from build123d import *

# Parameters (mm, degrees)
EXTRUDE006_DEPTH                          = 7.5
SKETCH004_R                               = 3.5
EXTRUDE005_DEPTH                          = 10
SKETCH003_AS_DRAWN_R                      = 2.05
EXTRUDE004_DEPTH                          = 4
EXTRUDE004_ONTO_SKETCH003_PLACEMENT_ANGLE = 25.679232
SKETCH002_AS_DRAWN_R                      = 2.05
EXTRUDE003_DEPTH                          = 4
EXTRUDE003_ONTO_SKETCH002_PLACEMENT_ANGLE = 25.679232
EXTRUDE002_DEPTH                          = 3
EXTRUDE001_DEPTH                          = 3
EXTRUDE_DEPTH                             = 100


with BuildPart() as extrude006:
    # Sketch005 (on Face9 of Cut002) → Extrude006 (new body, symmetric)
    with BuildSketch(Plane.XY.offset(-2.969462)):
        Polygon((9.788822, -17.287546), (13.381697, -21.769908), (23.066011, -14.007366), (19.473136, -9.525003), align=None)
        Polygon((74.935691, -52.555563), (78.706554, -57.139857), (89.207015, -48.502584), (85.436152, -43.91829), align=None)
        Polygon((9.274179, -44.439739), (14.585862, -39.004322), (26.329694, -50.48081), (21.018012, -55.916228), align=None)
        Polygon((69.684992, -9.981081), (73.170384, -6.034964), (84.857305, -16.35739), (81.371913, -20.303507), align=None)
    extrude(amount=EXTRUDE006_DEPTH, both=True)


with BuildPart() as extrude005:
    # Sketch004 (on Face13 of Cut001) → Extrude005 (new body, symmetric)
    with BuildSketch(Plane(origin=(0, 2.547184, 0), x_dir=(-1, 0, 0), z_dir=(0, 1, 0))):
        with Locations((-25.011261, 6.853597)):
            Circle(SKETCH004_R)
    extrude(amount=EXTRUDE005_DEPTH, both=True)


with BuildPart() as extrude004:
    # Sketch003 as drawn → Extrude004 (new)
    with BuildSketch(Plane.XY):
        with Locations((6.469403, -53.574993)):
            Circle(SKETCH003_AS_DRAWN_R)
        with Locations((93.253448, -53.665895)):
            Circle(SKETCH003_AS_DRAWN_R)
    extrude(amount=-EXTRUDE004_DEPTH)


with BuildPart() as extrude004_1:
    # Extrude004 onto Sketch003 placement: moved
    add(extrude004.part.moved(Location((0, -14.53972, 30.239351))).rotate(Axis((0, -14.53972, 30.239351), (1, 0, 0)), EXTRUDE004_ONTO_SKETCH003_PLACEMENT_ANGLE))


with BuildPart() as extrude003:
    # Sketch002 as drawn → Extrude003 (new)
    with BuildSketch(Plane.XY):
        with Locations((7.867664, 15.865227)):
            Circle(SKETCH002_AS_DRAWN_R)
        with Locations((92.333176, 15.993219)):
            Circle(SKETCH002_AS_DRAWN_R)
    extrude(amount=-EXTRUDE003_DEPTH)


with BuildPart() as extrude003_1:
    # Extrude003 onto Sketch002 placement: moved
    add(extrude003.part.moved(Location((0, -14.53972, 30.239351))).rotate(Axis((0, -14.53972, 30.239351), (1, 0, 0)), EXTRUDE003_ONTO_SKETCH002_PLACEMENT_ANGLE))


with BuildPart() as extrude002:
    # Sketch001 → Extrude002 (new body)
    with BuildSketch(Plane.YZ):
        Polygon((-59.93153, 8.316114), (-59.93153, -2.969465), (-2.952637, -2.969465), (-2.952637, 35.810581), align=None)
    extrude(amount=EXTRUDE002_DEPTH)


with BuildPart() as extrude002_1:
    # Extrude002 placement: moved
    add(extrude002.part.moved(Location((97, 0, 0))))


with BuildPart() as extrude001:
    # Sketch001 → Extrude001 (new body)
    with BuildSketch(Plane.YZ):
        Polygon((-59.93153, 8.316114), (-59.93153, -2.969465), (-2.952637, -2.969465), (-2.952637, 35.810581), align=None)
    extrude(amount=EXTRUDE001_DEPTH)


with BuildPart() as caja:
    # Sketch → Extrude (new body)
    with BuildSketch(Plane.YZ):
        Polygon((-65.452816, 5.759257), (-65.452816, -5.969462), (2.547184, -5.969462), (2.547184, 38.455096), (-2.952816, 35.81058), (-2.952816, -2.969462), (-59.952816, -2.969462), (-59.952816, 8.403773), align=None)
    extrude(amount=EXTRUDE_DEPTH)

    # Fusion: union Extrude002, Extrude001
    add(extrude002_1.part)
    add(extrude001.part)

    # Cut: cut Extrude003
    add(extrude003_1.part, mode=Mode.SUBTRACT)

    # Cut001: cut Extrude004
    add(extrude004_1.part, mode=Mode.SUBTRACT)

    # Cut002: cut Extrude005
    add(extrude005.part, mode=Mode.SUBTRACT)

    # Cut003: cut Extrude006
    add(extrude006.part, mode=Mode.SUBTRACT)


solid = caja.part
Can you work these out from the model? Positions are in its coordinate system, mm. A direction names the side the tool comes from. Give positions to 0.01 mm unless a question says otherwise; leave off trailing zeros. Order: outer loops, then holes, each group sorted by start corner. A loop starts at its lowest first (then second) coordinate and runs counter-clockwise, first axis right, second up. Notation, with made-up numbers: M 25,32.5 L 72,32.5 A28 cw 72,69.5 Z; hole C -35.75,67 d7. An arc over 180 degrees is marked long. One line per item, written item: value.
Item 1: If we section it at C-C on x = 30: Write out the boundary of the cut face in (y, z).
Verdict:
outline: M -65.45,-5.97 L 2.55,-5.97 L 2.55,38.46 L -2.95,35.81 L -2.95,-2.97 L -59.95,-2.97 L -59.95,8.4 L -65.45,5.76 Z
Item 2: Please list where these lines run through material, in increasing order: line 1 (X direction, y = -23.5, z = 20); line 2 (Y direction, x = 16, z = 0); line 3 (X direction, y = -12.5, z = -3).
Verdict:
line 1: 0 to 3, 97 to 100
line 2: -65.45 to -59.95, -2.95 to 2.55
line 3: 0 to 15.76, 21.86 to 72.54, 80.49 to 100
Item 3: For pin 1 (4 mm diameter, centred on x = 24.5, z = 19.5, fed in from -Y); pin 2 (11.5 mm diameter, centred on x = 44.5, z = 14, fed in from -Y), each with a flat end and sliding along its axis, tell me the tip position at first contact or that it passes through.
Verdict:
pin 1: y = -2.95
pin 2: y = -60.27
Item 4: For faces 1 (the face through (92.304, 1.173, 33.356)), 2 (the face through (49, -2.953, 17)), 3 (the face through (20.376, -44.662, -4.49)), 4 (the face through (1.479, -31.043, 22.256)), which set-ups out of +Z, -Z, +X, -X, +Y, -Y let a thin tool reach every point of the face, with its end or its side?
Verdict:
face 1: none
face 2: +Z
face 3: +Z, -Z
face 4: +Z, +X, -X, -Y
Item 5: If we section it at B-B on y = -8: Write out the boundary of the cut face in (x, z).
Verdict:
outline: M 0,-5.97 L 71.43,-5.97 L 71.43,-2.97 L 3,-2.97 L 3,33.38 L 0,33.38 Z; M 75.4,-5.97 L 100,-5.97 L 100,33.38 L 97,33.38 L 97,-2.97 L 75.4,-2.97 Z
Item 6: If we section it at A-A on z = -0.5: Write out the boundary of the cut face in (x, y).
Verdict:
outline: M 0,-65.45 L 100,-65.45 L 100,-59.95 L 0,-59.95 Z; M 0,-59.93 L 3,-59.93 L 3,-2.95 L 97,-2.95 L 97,-59.93 L 100,-59.93 L 100,2.55 L 0,2.55 Z
Item 7: If we mould it in two halves opening along X, with no side actions, what happens to faces 5 (the face through (100, -24, 12)), 6 (the face through (11.893, -41.76, -4.49)), 7 (the face through (49.3, -62.66, 7.1))? For each: pulls with the +X half, pulls with the -X half, needs draft (parallel to the pull), parting line crosses it, or undercut.
Verdict:
face 5: pulls with the +X half
face 6: undercut
face 7: needs draft
Item 8: If we section it at D-D on z = 11.5: Write out the boundary of the cut face in (x, y).
Verdict:
outline: M 0,-53.33 L 3,-53.33 L 3,-2.95 L 97,-2.95 L 97,-53.33 L 100,-53.33 L 100,2.55 L 0,2.55 Z
